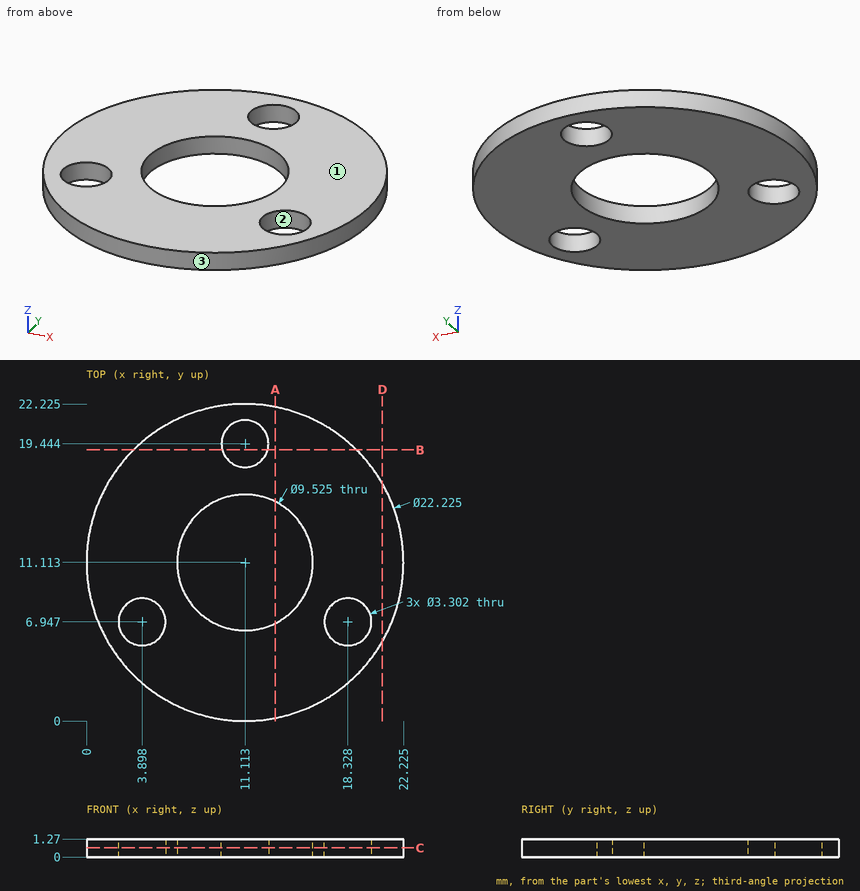
Here's the drawing with two shaded views (mm, measured from the low corner). I have some questions. Give positions to 0.01 mm unless a question says otherwise; leave off trailing zeros. Loops run counter-clockwise (first coordinate to the right, second up) from the corner with the lowest first, then second, coordinate; pieces in that order, holes last. Notation, with made-up numbers: M 49,-20.75 L 79,-20.75 A14 ccw 79,-5.75 Z; hole C 32,-23 d8. An arc over 180 degrees is marked long. Use one line per item in the form item = value. Start each with the question number.
Q1. If we section it at D-D (x = 20.75): Write out the boundary of the cut face in (y, z) (1 decimal).
Q2. If we section it at C-C (z = 0.65): State how many separate pieces and enclosed holes the cut face has, then the cut area to 3 significant figures.
Q3. If we section it at A-A (x = 13.25): Write out the boundary of the cut face in (y, z), then the cut area to 3 significant figures.
Q4. I need wall thicknesses on line 1 along X through (y, z) = (8, 0.1) (1 decimal); line 2 along X through (y, z) = (5.5, 0.8) (1 decimal); line 3 along Y through (x, z) = (14.5, 1.05) (1 decimal). Which ranges of each line are inside material? Lowest first, please.
Q5. Thinking about a two-plate mould opening in Y: for the marked faces 1, 2 and 3, which applies, +Y half, -Y half, draft (parallel to the pull), parting line (faces both ways), or undercut?
Q6. If we section it at B-B (y = 19): Write out the boundary of the cut face in (x, z) (1 decimal).
Taken from the geometry:
q1.outline = M 5.6,0 L 16.6,0 L 16.6,1.3 L 5.6,1.3 Z
q2.separate_pieces = 1
q2.enclosed_holes = 4
q2.area = 291 mm^2
q3.outline = M 0.21,0 L 6.86,0 L 6.86,1.27 L 0.21,1.27 Z; M 15.37,0 L 22.02,0 L 22.02,1.27 L 15.37,1.27 Z
q3.area = 16.9 mm^2
q4.line_1 = 0.4 to 2.6, 5.2 to 7.5, 14.7 to 17.1, 19.6 to 21.8
q4.line_2 = 1.5 to 3.1, 4.7 to 17.5, 19.1 to 20.7
q4.line_3 = 0.5 to 7.8, 14.5 to 21.7
q5.face_1 = draft
q5.face_2 = undercut
q5.face_3 = parting line
q6.outline = M 3.3,0 L 9.5,0 L 9.5,1.3 L 3.3,1.3 Z; M 12.7,0 L 18.9,0 L 18.9,1.3 L 12.7,1.3 Z
